Check sheet for the modelled part. Datum: model origin and axes. Units: mm. A direction names the side the tool comes from. Round coordinates to 2 decimals unless told otherwise and drop trailing zeros. Order: outer loops, then holes, each group sorted by start corner. A loop starts at its lowest first (then second) coordinate and runs counter-clockwise, first axis right, second up. Notation, with made-up numbers: (14, -17.5) -> (29, -17.5) arc R21 ccw to (29, 11.5) -> close; hole circle Ø4 at (20, 4). An arc over 180 degrees is marked (long way). Answer in a Markdown table with one row per item.
from build123d import *

# Parameters (mm, degrees)
F0_R     = 12.5
F3_DEPTH = 5
F1_R     = 2.5
F4_DEPTH = 10
F2_R     = 2.5
F6_DEPTH = 3
F7_R     = 5.046872
F8_DEPTH = 10


with BuildPart() as f3:
    # F0 (on Right) → F3 (new body)
    with BuildSketch(Plane.YZ):
        Circle(F0_R)
    extrude(amount=F3_DEPTH)

    # F1 (on Right) → F4 (cut)
    with BuildSketch(Plane.YZ):
        Circle(F1_R)
    extrude(amount=F4_DEPTH, mode=Mode.SUBTRACT)

    # F2 (on Right) → F6 (cut)
    with BuildSketch(Plane.YZ):
        Circle(F2_R)
    extrude(amount=F6_DEPTH, mode=Mode.SUBTRACT)

    # F7 (on face) → F8 (join)
    with BuildSketch(Plane.YZ):
        Circle(F7_R)
    extrude(amount=-F8_DEPTH)


solid = f3.part
Item 1: Cross-section at D-D (x = -5). Record the boundary of the cut face in (y, z), and give its area (3 significant figures).
Result sheet:
| item | result |
|---|---|
| outline | circle Ø10.09 at (0, 0) |
| area | 80.0 mm^2 |
Item 2: Cross-section at B-B (x = 3.25). Record the boundary of the cut face in (y, z).
Result sheet:
| item | result |
|---|---|
| outline | circle Ø25 at (0, 0); hole circle Ø5 at (0, 0) |
Item 3: Mould release check, pull along Z, two halves, no side actions. Record for faces 4 (the flat face through (5, 0, -3)), 5 (the flat face through (0, 0, 0)), 6 (the cylindrical face through (-4.93, 4.814, 1.516)): pulls with the +Z half, pulls with the -Z half, needs draft (parallel to the pull), parting line crosses it, or undercut.
Result sheet:
| item | result |
|---|---|
| face 4 | needs draft |
| face 5 | undercut |
| face 6 | parting line crosses it |
Item 4: Cross-section at A-A (z = 0). Record the boundary of the cut face in (x, y).
Result sheet:
| item | result |
|---|---|
| outline | (-10, -5.05) -> (0, -5.05) -> (0, -12.5) -> (5, -12.5) -> (5, -2.5) -> (0, -2.5) -> (0, 2.5) -> (5, 2.5) -> (5, 12.5) -> (0, 12.5) -> (0, 5.05) -> (-10, 5.05) -> close |
Item 5: Scan lines: line 1 (Z direction, x = 3.4, y = 0); line 2 (X direction, y = 8.25, z = -2.25); line 3 (X direction, y = 1.25, z = 1.5). Record each from-to range of solid material in increasing order. Write a range as [from, to].
Result sheet:
| item | result |
|---|---|
| line 1 | z = [-12.5, -2.5], [2.5, 12.5] |
| line 2 | x = [0, 5] |
| line 3 | x = [-10, 0] |
Item 6: Set-up check for faces 1 (the cylindrical face through (2.46, -0.54, -2.44)), 2 (the flat face through (0, -0.2, -5.4)), 3 (the cylindrical face through (2.465, 11.923, 3.755)): record each of +Z, -Z, +X, -X, +Y, -Y from which the full face is reachable in a straight line by a thin tool's end or side.
Result sheet:
| item | result |
|---|---|
| face 1 | +X |
| face 2 | -X |
| face 3 | +X, -X |
Item 7: Depth check by flat-ended pin: P1, Ø2.5, axis at y = 0, z = 0, coming from the +X side; P2, Ø1, axis at x = 3, y = -8, coming from the -Z side; P3, Ø4, axis at y = -1, z = 10, coming from the -X side. Enter the tip coordinate at first touch or a pass-through.
Result sheet:
| item | result |
|---|---|
| P1 | stops at x = 0 |
| P2 | stops at z = -10 |
| P3 | stops at x = 0 |
